```python
from build123d import *

# Parameters (mm, degrees)
SKETCH1_W           = 120
SKETCH1_H           = 70
SKETCH1_R           = 3
SKETCH1_W_2         = 12
SKETCH1_H_2         = 46
BOSS_EXTRUDE1_DEPTH = 7.2
FILLET1_R           = 2
SKETCH2_W           = 120
SKETCH2_H           = 5
BOSS_EXTRUDE2_DEPTH = 70
SKETCH3_W           = 7.2
SKETCH3_H           = 60
BOSS_EXTRUDE3_DEPTH = 50
SKETCH4_R           = 4
SKETCH4_R_2         = 1.5
CUT_EXTRUDE1_DEPTH  = 10
SKETCH5_R           = 8.5
CUT_EXTRUDE2_DEPTH  = 3
SKETCH6_W           = 7.2
SKETCH6_H           = 60
BOSS_EXTRUDE4_DEPTH = 55
CUT_EXTRUDE4_DEPTH  = 4
CUT_EXTRUDE5_START  = -60
SKETCH10_R          = 4
CUT_EXTRUDE5_DEPTH  = 60
SKETCH11_R          = 19.175
CUT_EXTRUDE6_DEPTH  = 7.2


with BuildPart() as part:
    # Sketch1 → Boss-Extrude1 (new body)
    with BuildSketch(Plane(origin=(0, 0, 0), x_dir=(1, 0, 0), z_dir=(0, 1, 0))):
        Rectangle(SKETCH1_W, SKETCH1_H)
        with Locations(Location((-37.5, 24, 0), (0, 0, 270))):
            Circle(SKETCH1_R, mode=Mode.SUBTRACT)
        with Locations(Location((-37.5, -24, 0), (0, 0, 90))):
            Circle(SKETCH1_R, mode=Mode.SUBTRACT)
        with Locations(Location((37.5, 24, 0), (0, 0, 90))):
            Circle(SKETCH1_R, mode=Mode.SUBTRACT)
        with Locations(Location((37.5, -24, 0), (0, 0, 270))):
            Circle(SKETCH1_R, mode=Mode.SUBTRACT)
        Rectangle(SKETCH1_W_2, SKETCH1_H_2, mode=Mode.SUBTRACT)
    extrude(amount=BOSS_EXTRUDE1_DEPTH)

    # Fillet1
    fillet1_edges = [part.edges().sort_by_distance(p)[0] for p in [
        (-6, 3.6, -23),
        (-6, 3.6, 23),
        (6, 3.6, 23),
        (6, 3.6, -23),
    ]]
    fillet(fillet1_edges, radius=FILLET1_R)

    # Sketch2 → Boss-Extrude2 (add)
    with BuildSketch(Plane.XZ):
        with Locations((0, -32.5)):
            Rectangle(SKETCH2_W, SKETCH2_H)
    extrude(amount=BOSS_EXTRUDE2_DEPTH)

    # Sketch3 → Boss-Extrude3 (add)
    with BuildSketch(Plane.XY.offset(-30)):
        with Locations((-9.6, -30)):
            Rectangle(SKETCH3_W, SKETCH3_H)
    extrude(amount=BOSS_EXTRUDE3_DEPTH)

    # Sketch4 → Cut-Extrude1 (cut)
    with BuildSketch(Plane.ZY.offset(13.2)):
        with Locations((0, -30)):
            Circle(SKETCH4_R)
        with Locations((0, -19)):
            Circle(SKETCH4_R_2)
        with Locations((-9.526279442, -24.5)):
            Circle(SKETCH4_R_2)
        with Locations((-9.526279442, -35.5)):
            Circle(SKETCH4_R_2)
        with Locations((0, -41)):
            Circle(SKETCH4_R_2)
        with Locations((9.526279442, -35.5)):
            Circle(SKETCH4_R_2)
        with Locations((9.526279442, -24.5)):
            Circle(SKETCH4_R_2)
    extrude(amount=-CUT_EXTRUDE1_DEPTH, mode=Mode.SUBTRACT)

    # Sketch5 → Cut-Extrude2 (cut)
    with BuildSketch(Plane.ZY.offset(13.2)):
        with Locations((0, -30)):
            Circle(SKETCH5_R)
    extrude(amount=-CUT_EXTRUDE2_DEPTH, mode=Mode.SUBTRACT)

    # Sketch6 → Boss-Extrude4 (add)
    with BuildSketch(Plane.XY.offset(-30)):
        with Locations((-56.4, -30)):
            Rectangle(SKETCH6_W, SKETCH6_H)
    extrude(amount=BOSS_EXTRUDE4_DEPTH)

    # Sketch8 → Cut-Extrude4 (cut)
    with BuildSketch(Plane.XZ):
        Polygon((42.7, 27.0022214), (37.5, 30.0044428), (32.3, 27.0022214), (32.3, 20.9977786), (37.5, 17.9955572), (42.7, 20.9977786), align=None)
        Polygon((-32.3, 27.0022214), (-37.5, 30.0044428), (-42.7, 27.0022214), (-42.7, 20.9977786), (-37.5, 17.9955572), (-32.3, 20.9977786), align=None)
        Polygon((42.7, -20.9977786), (37.5, -17.9955572), (32.3, -20.9977786), (32.3, -27.0022214), (37.5, -30.0044428), (42.7, -27.0022214), align=None)
        Polygon((-32.3, -20.9977786), (-37.5, -17.9955572), (-42.7, -20.9977786), (-42.7, -27.0022214), (-37.5, -30.0044428), (-32.3, -27.0022214), align=None)
    extrude(amount=-CUT_EXTRUDE4_DEPTH, mode=Mode.SUBTRACT)

    # Sketch10 → Cut-Extrude5 (cut)
    with BuildSketch(Plane(origin=(-6, 0, 0), x_dir=(0, 0, -1), z_dir=(1, 0, 0)).offset(CUT_EXTRUDE5_START)):
        with Locations(Location((0, -30, 0), (0, 0, 180))):
            Circle(SKETCH10_R)
    extrude(amount=CUT_EXTRUDE5_DEPTH, mode=Mode.SUBTRACT)

    # Sketch11 → Cut-Extrude6 (cut)
    with BuildSketch(Plane.ZY.offset(60)):
        with Locations((0, -30)):
            Circle(SKETCH11_R)
    extrude(amount=-CUT_EXTRUDE6_DEPTH, mode=Mode.SUBTRACT)


solid = part.part
```
The listing builds one solid part. Answer for the finished solid, in the listing's coordinates (mm). A direction names the side the tool comes from. Round coordinates to 2 decimals unless told otherwise and drop trailing zeros. Order: outer loops, then holes, each group sorted by start corner. A loop starts at its lowest first (then second) coordinate and runs counter-clockwise, first axis right, second up. Notation, with made-up numbers: (-29.5, 58) -> (-22.5, 58) arc R17 ccw to (-22.5, 62) -> close; hole circle Ø3 at (-39.75, -27.75). An arc over 180 degrees is marked (long way). Answer as CSV lines item,"result".
Q1. Consider line 1 (Z direction, x = -37.5, y = 5.35); line 2 (X direction, y = 5, z = 24); line 3 (X direction, y = -26.5, z = -25). Determine where each line is inside the solid, lowest interval first. Write a range as from..to.
Computed values:
line 1,"z = -35..-27, -21..21, 27..35"
line 2,"x = -60..-40.5, -34.5..34.5, 40.5..60"
line 3,"x = -60..-52.8, -13.2..-6"
Q2. A cutting plane is placed at B-B on z = -16. Determine the outline of the cut face in (x, y), plus the area to 3 significant figures.
Computed values:
outline,"(-60, -60) -> (-52.8, -60) -> (-52.8, -40.57) -> (-60, -40.57) -> close; (-60, -19.43) -> (-52.8, -19.43) -> (-52.8, 0) -> (-13.2, 0) -> (-13.2, -60) -> (-6, -60) -> (-6, 7.2) -> (-60, 7.2) -> close; (6, 0) -> (60, 0) -> (60, 7.2) -> (6, 7.2) -> close"
area,"1,490 mm^2"
Q3. For a pull along X with two mould halves and no side action, classify faces 5 (the cylindrical face through (-56.45, -10.99, -2.5)), 6 (the flat face through (-40.064, 1.972, 28.524)) as +X half, -X half, draft (parallel to the pull), parting line (faces both ways), or undercut.
Computed values:
face 5,"draft"
face 6,"undercut"
Q4. Which of the six approach directions +Z, -Z, +X, -X, +Y, -Y give full straight-line access (tool end or side, diameter ignored) to faces 1 (the flat face through (-32.3, 2, -24)), 2 (the flat face through (-56, -60, -3)), 3 (the flat face through (0, 4, -23)), 4 (the cylindrical face through (-11.72, -38.3, -1.84))?
Computed values:
face 1,"-Y"
face 2,"+Z, +X, -X, -Y"
face 3,"+Y, -Y"
face 4,"-X"
Q5. A cutting plane is placed at C-C on y = -5.5. Determine the outline of the cut face in (x, z).
Computed values:
outline,"(-60, -35) -> (60, -35) -> (60, -30) -> (-6, -30) -> (-6, 20) -> (-13.2, 20) -> (-13.2, -30) -> (-52.8, -30) -> (-52.8, 25) -> (-60, 25) -> close"
Q6. Given pin 1 (1.5 mm diameter, centred on x = -40.5, y = -50, fed in from +Z); pin 2 (13.5 mm diameter, centred on y = -30, z = 0, fed in from -X); pin 3 (6 mm diameter, centred on x = 15.5, z = -13, fed in from -Y), each flat-ended and moving along its own axis, determine where each tip first touches the part or whether it passes through.
Computed values:
pin 1,"stops at z = -30"
pin 2,"stops at x = -10.2"
pin 3,"stops at y = 0"
Q7. A cutting plane is placed at A-A on y = -24.5. Determine the outline of the cut face in (x, z), plus the area to 3 significant figures.
Computed values:
outline,"(-60, -35) -> (60, -35) -> (60, -30) -> (-6, -30) -> (-6, -11.03) -> (-13.2, -11.03) -> (-13.2, -30) -> (-52.8, -30) -> (-52.8, -18.37) -> (-60, -18.37) -> close; (-60, 18.37) -> (-52.8, 18.37) -> (-52.8, 25) -> (-60, 25) -> close; (-13.2, -8.03) -> (-6, -8.03) -> (-6, 8.03) -> (-13.2, 8.03) -> (-13.2, 6.48) -> (-10.2, 6.48) -> (-10.2, -6.48) -> (-13.2, -6.48) -> close; (-13.2, 11.03) -> (-6, 11.03) -> (-6, 20) -> (-13.2, 20) -> close"
area,"1,010 mm^2"
Q8. A cutting plane is placed at D-D on x = 45. Determine the outline of the cut face in (y, z), plus the area to 3 significant figures.
Computed values:
outline,"(-70, -35) -> (7.2, -35) -> (7.2, 35) -> (0, 35) -> (0, -30) -> (-70, -30) -> close"
area,"854 mm^2"
